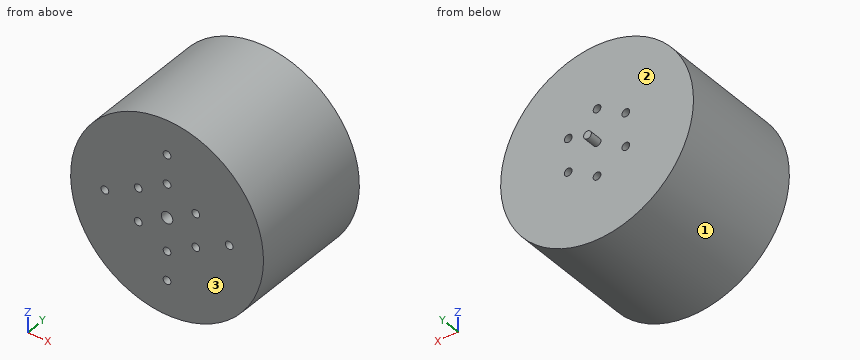
```python
from build123d import *

# Parameters (mm, degrees)
SKETCH_1_R          = 50
EXTRUDE_1_DEPTH     = 66
SKETCH_2_R          = 2
CUT_EXTRUDE_2_DEPTH = 97.726418315
SKETCH_3_R          = 2
EXTRUDE_2_DEPTH     = 6.6
SKETCH_4_R          = 3
CUT_EXTRUDE_3_DEPTH = 6
SKETCH_8_R          = 2
CUT_EXTRUDE_4_DEPTH = 6


with BuildPart() as part:
    # 草图1 → 凸台-拉伸1 (new body)
    with BuildSketch(Plane(origin=(0, 0, 0), x_dir=(1, 0, 0), z_dir=(0, 1, 0))):
        with Locations(Location((0, 0, 0), (0, 0, 270))):
            Circle(SKETCH_1_R)
    extrude(amount=EXTRUDE_1_DEPTH)

    # 草图2 → 切除-拉伸2 (cut, through all)
    with BuildSketch(Plane(origin=(0, 66, 0), x_dir=(1, 0, 0), z_dir=(0, 1, 0))):
        with Locations(Location((0, 17.25, 0), (0, 0, 270))):
            Circle(SKETCH_2_R)
        with Locations(Location((14.938938215, 8.625, 0), (0, 0, 270))):
            Circle(SKETCH_2_R)
        with Locations(Location((14.938938215, -8.625, 0), (0, 0, 270))):
            Circle(SKETCH_2_R)
        with Locations(Location((0, -17.25, 0), (0, 0, 270))):
            Circle(SKETCH_2_R)
        with Locations(Location((-14.938938215, -8.625, 0), (0, 0, 270))):
            Circle(SKETCH_2_R)
        with Locations(Location((-14.938938215, 8.625, 0), (0, 0, 270))):
            Circle(SKETCH_2_R)
    extrude(amount=-CUT_EXTRUDE_2_DEPTH, mode=Mode.SUBTRACT)

    # 草图3 → 凸台-拉伸2 (add)
    with BuildSketch(Plane(origin=(0, 66, 0), x_dir=(1, 0, 0), z_dir=(0, 1, 0))):
        with Locations(Location((0, 0, 0), (0, 0, 270))):
            Circle(SKETCH_3_R)
    extrude(amount=EXTRUDE_2_DEPTH)

    # 草图4 → 切除-拉伸3 (cut)
    with BuildSketch(Plane(origin=(0, 0, 0), x_dir=(-1, 0, 0), z_dir=(0, -1, 0))):
        with Locations(Location((0, 0, 0), (0, 0, 90))):
            Circle(SKETCH_4_R)
    extrude(amount=-CUT_EXTRUDE_3_DEPTH, mode=Mode.SUBTRACT)

    # 草图8 → 切除-拉伸4 (cut)
    with BuildSketch(Plane(origin=(0, 0, 0), x_dir=(-1, 0, 0), z_dir=(0, -1, 0))):
        with Locations(Location((0, 32.222894459, 0), (0, 0, 90))):
            Circle(SKETCH_8_R)
        with Locations(Location((32.222894459, 0, 0), (0, 0, 90))):
            Circle(SKETCH_8_R)
        with Locations(Location((0, -32.222894459, 0), (0, 0, 90))):
            Circle(SKETCH_8_R)
        with Locations(Location((-32.222894459, 0, 0), (0, 0, 90))):
            Circle(SKETCH_8_R)
    extrude(amount=-CUT_EXTRUDE_4_DEPTH, mode=Mode.SUBTRACT)


solid = part.part
```
The model under review builds one solid part; all positions refer to its coordinate system, in mm. Face numbers are marked on the shaded views. Round coordinates to 2 decimals unless told otherwise and drop trailing zeros. Loops run counter-clockwise (first coordinate to the right, second up) from the corner with the lowest first, then second, coordinate; pieces in that order, holes last. Notation, with made-up numbers: (-11.5, 59.25) -> (-3.5, 59.25) arc R31 cw to (-3.5, 87.25) -> close; hole circle Ø10 at (56.5, -32.75). An arc over 180 degrees is marked (long way). Answer in a Markdown table with one row per item.
1) For pin 1 Ø2.5 at (x, z) = (-14.94, -8.62) entering from -Y; pin 2 Ø3 at (y, z) = (61.5, -39.5) entering from +X; pin 3 Ø1 at (x, y) = (-33.5, 21.5) entering from -Z; pin 4 Ø4.5 at (x, z) = (0, 17.25) entering from +Y, all flat-tipped, find the tip position at first contact; note any pin that passes through.
Taken from the geometry:
| item | result |
|---|---|
| pin 1 | passes through |
| pin 2 | stops at x = 32.5 |
| pin 3 | stops at z = -37.56 |
| pin 4 | stops at y = 66 |
2) Consider section A-A, the plane x = 0. Write out the cut boundary in (y, z), plus the area to 3 significant figures.
Taken from the geometry:
| item | result |
|---|---|
| outline | (0, -50) -> (66, -50) -> (66, -19.25) -> (0, -19.25) -> (0, -30.22) -> (6, -30.22) -> (6, -34.22) -> (0, -34.22) -> close; (0, -15.25) -> (66, -15.25) -> (66, -2) -> (72.6, -2) -> (72.6, 2) -> (66, 2) -> (66, 15.25) -> (0, 15.25) -> (0, 3) -> (6, 3) -> (6, -3) -> (0, -3) -> close; (0, 19.25) -> (66, 19.25) -> (66, 50) -> (0, 50) -> (0, 34.22) -> (6, 34.22) -> (6, 30.22) -> (0, 30.22) -> close |
| area | 6,010 mm² |
3) Draft analysis for pull direction Y (two halves, no side actions). For the marked faces 1, 2 and 3, state which applies: pulls with the +Y half, pulls with the -Y half, needs draft (parallel to the pull), parting line crosses it, or undercut.
Taken from the geometry:
| item | result |
|---|---|
| face 1 | needs draft |
| face 2 | pulls with the +Y half |
| face 3 | pulls with the -Y half |
4) Consider section D-D, the plane y = 26.5. Write out the cut boundary in (x, z) (3 decimals).
Taken from the geometry:
| item | result |
|---|---|
| outline | circle Ø100 at (0, 0); hole circle Ø4 at (-14.939, -8.625); hole circle Ø4 at (-14.939, 8.625); hole circle Ø4 at (0, -17.25); hole circle Ø4 at (0, 17.25); hole circle Ø4 at (14.939, -8.625); hole circle Ø4 at (14.939, 8.625) |
5) Consider section C-C, the plane z = 0. Write out the cut boundary in (x, y).
Taken from the geometry:
| item | result |
|---|---|
| outline | (-50, 0) -> (-34.22, 0) -> (-34.22, 6) -> (-30.22, 6) -> (-30.22, 0) -> (-3, 0) -> (-3, 6) -> (3, 6) -> (3, 0) -> (30.22, 0) -> (30.22, 6) -> (34.22, 6) -> (34.22, 0) -> (50, 0) -> (50, 66) -> (2, 66) -> (2, 72.6) -> (-2, 72.6) -> (-2, 66) -> (-50, 66) -> close |
6) Consider section B-B, the plane z = 17.25. Write out the cut boundary in (x, y).
Taken from the geometry:
| item | result |
|---|---|
| outline | (-46.93, 0) -> (-2, 0) -> (-2, 66) -> (-46.93, 66) -> close; (2, 0) -> (46.93, 0) -> (46.93, 66) -> (2, 66) -> close |
7) Wall thickness on line 1 along X through (y, z) = (2, 0); line 2 along Y through (x, z) = (-12.5, 44); line 3 along Z through (x, y) = (-1, 42): over which ranges is each line inside the solid? List them lowest first.
Taken from the geometry:
| item | result |
|---|---|
| line 1 | x = -50 to -34.22, -30.22 to -3, 3 to 30.22, 34.22 to 50 |
| line 2 | y = 0 to 66 |
| line 3 | z = -49.99 to -18.98, -15.52 to 15.52, 18.98 to 49.99 |
